Answer from the drawing. Dimensions are ordinates in mm from the lowest x, y and z of the part. Round coordinates to 2 decimals unless told otherwise and drop trailing zeros. Write each loop counter-clockwise with the first axis right and the second up, starting at its lowest first coordinate (ties: lowest second). Pieces come first, ordered by that corner, then holes. Notation, with made-up numbers: (52, 30) - (94, 30) arc R14 cw to (94, 38) - close; hole circle Ø5 at (59, -9.75). An arc over 180 degrees is marked (long way). Answer as a JSON object with one key per item and string values.
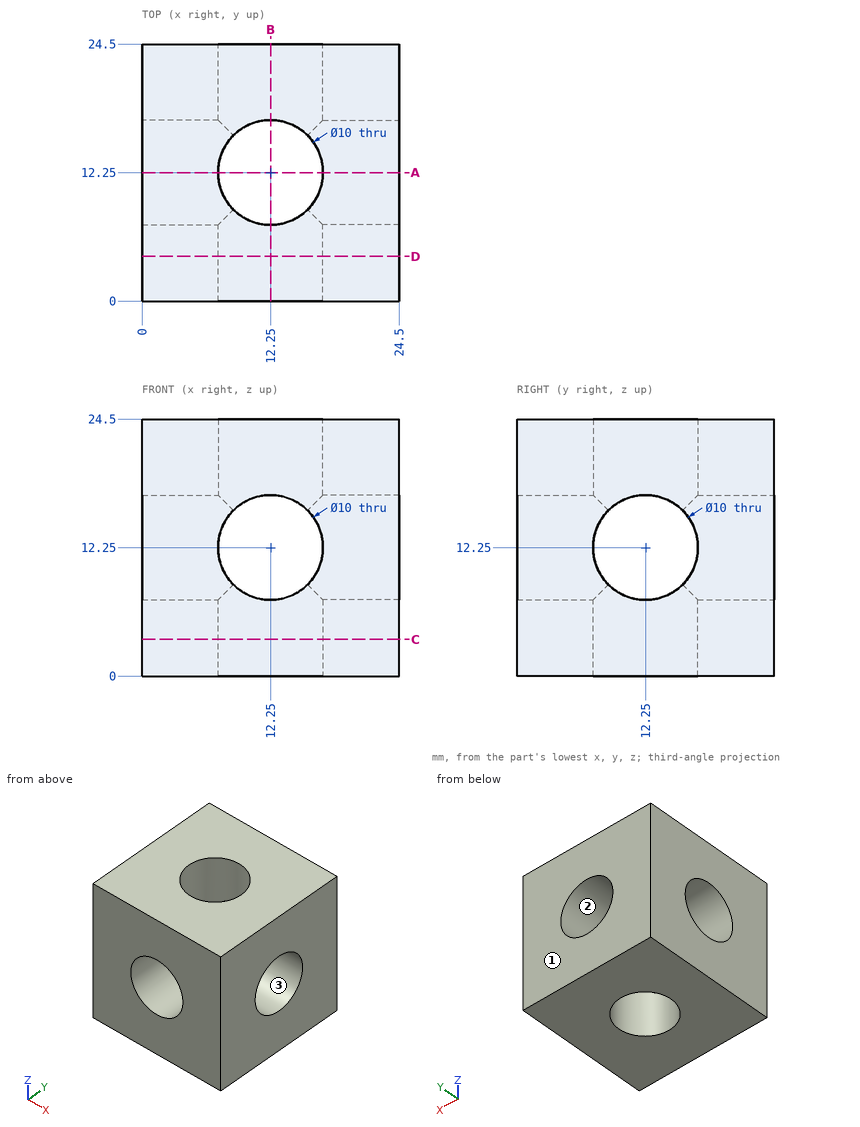
Item 1: Determine the mould class of the marked faces 1, 2 and 3 for opening direction Y: pulls with the +Y half, pulls with the -Y half, needs draft (parallel to the pull), parting line crosses it, or undercut.
Results found:
{"face 1": "pulls with the +Y half", "face 2": "needs draft", "face 3": "undercut"}
Item 2: A cutting plane is placed at C-C (z = 3.5). Write down the section's boundary in (x, y), and give its area (3 significant figures).
Results found:
{"outline": "(0, 0) - (24.5, 0) - (24.5, 24.5) - (0, 24.5) - close; hole circle Ø10 at (12.25, 12.25)", "area": "522 mm²"}
Item 3: This flat-tipped pin is pushed along its axis until it touches: P1, Ø6, axis at x = 12.25, y = 12.25, coming from the +Z side. Where does it stop, or does it pass through?
Results found:
{"P1": "through"}
Item 4: A cutting plane is placed at A-A (y = 12.25). Write down the section's boundary in (x, z).
Results found:
{"outline": "(0, 0) - (7.25, 0) - (7.25, 7.25) - (0, 7.25) - close; (0, 17.25) - (7.25, 17.25) - (7.25, 24.5) - (0, 24.5) - close; (17.25, 0) - (24.5, 0) - (24.5, 7.25) - (17.25, 7.25) - close; (17.25, 17.25) - (24.5, 17.25) - (24.5, 24.5) - (17.25, 24.5) - close"}
Item 5: Consider line 1 along Y through (x, z) = (12.25, 6). Determine where the line is inside the solid, lowest interval first.
Results found:
{"line 1": "0 to 7.25, 17.25 to 24.5"}
